```python
from build123d import *

# Parameters (mm, degrees)
F0_R     = 63.5
F0_R_2   = 1.5875
F1_DEPTH = 3.175


with BuildPart() as f1:
    # F0 (on Front) → F1 (new body)
    with BuildSketch(Plane.XZ):
        Circle(F0_R)
        with BuildLine():
            ThreePointArc((-12.832221, -55.690723), (-24.872502, -51.45368), (-35.672091, -44.650021))
            Line((-35.672091, -44.650021), (-8.873024, -9.086223))
            ThreePointArc((-8.873024, -9.086223), (-5.527223, -11.434151), (-1.608887, -12.597678))
            Line((-1.608887, -12.597678), (-12.832221, -55.690723))
        make_face(mode=Mode.SUBTRACT)
        with BuildLine():
            ThreePointArc((-51.541519, -24.689963), (-55.735858, -12.634739), (-57.149977, 0.050731))
            Line((-57.149977, 0.050731), (-12.636135, 1.272042))
            ThreePointArc((-12.636135, 1.272042), (-12.385746, -2.80772), (-10.852385, -6.596645))
            Line((-10.852385, -6.596645), (-51.541519, -24.689963))
        make_face(mode=Mode.SUBTRACT)
        with BuildLine():
            ThreePointArc((35.540001, -44.755232), (24.720355, -51.52695), (12.667607, -55.728397))
            Line((12.667607, -55.728397), (1.571655, -12.602377))
            ThreePointArc((1.571655, -12.602377), (5.493412, -11.450433), (8.846137, -9.112402))
            Line((8.846137, -9.112402), (35.540001, -44.755232))
        make_face(mode=Mode.SUBTRACT)
        with BuildLine():
            ThreePointArc((57.149878, -0.118139), (55.698281, -12.799376), (51.468339, -24.842153))
            Line((51.468339, -24.842153), (10.832846, -6.628684))
            ThreePointArc((10.832846, -6.628684), (12.377396, -2.844306), (12.639839, 1.234699))
            Line((12.639839, 1.234699), (57.149878, -0.118139))
        make_face(mode=Mode.SUBTRACT)
        with BuildLine():
            ThreePointArc((-51.439002, 24.902842), (-44.628976, 35.698417), (-35.592765, 44.713282))
            Line((-35.592765, 44.713282), (-6.883979, 10.672433))
            ThreePointArc((-6.883979, 10.672433), (-9.91755, 7.932982), (-11.923817, 4.371795))
            Line((-11.923817, 4.371795), (-51.439002, 24.902842))
        make_face(mode=Mode.SUBTRACT)
        Circle(F0_R_2, mode=Mode.SUBTRACT)
        with BuildLine():
            ThreePointArc((35.724731, 44.607915), (44.734265, 35.566389), (51.512362, 24.750739))
            Line((51.512362, 24.750739), (11.936683, 4.336543))
            ThreePointArc((11.936683, 4.336543), (9.940948, 7.903642), (6.915484, 10.652046))
            Line((6.915484, 10.652046), (35.724731, 44.607915))
        make_face(mode=Mode.SUBTRACT)
        with BuildLine():
            ThreePointArc((-12.601867, 55.7433), (0.084435, 57.149938), (12.766526, 55.705819))
            Line((12.766526, 55.705819), (4.051954, 12.036265))
            ThreePointArc((4.051954, 12.036265), (0.018763, 12.699986), (-4.016371, 12.048185))
            Line((-4.016371, 12.048185), (-12.601867, 55.7433))
        make_face(mode=Mode.SUBTRACT)
    extrude(amount=F1_DEPTH)


solid = f1.part
```
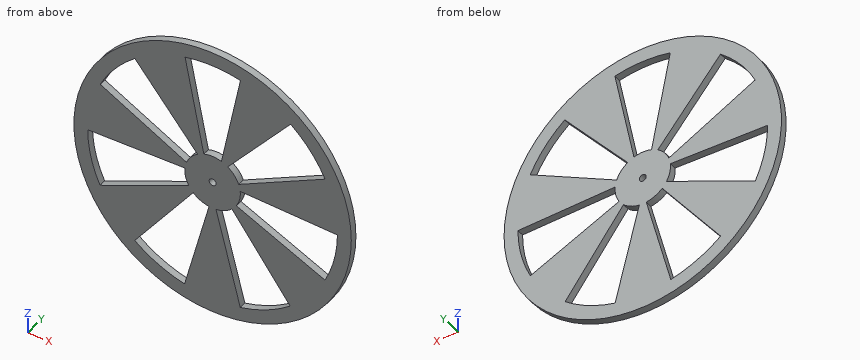
Work out the finished part from the listing and answer in its coordinate system (mm). Round coordinates to 2 decimals unless told otherwise and drop trailing zeros. Write each loop counter-clockwise with the first axis right and the second up, starting at its lowest first coordinate (ties: lowest second). Pieces come first, ordered by that corner, then holes.
1) A cutting plane is placed at B-B on z = 18. Determine the outline of the cut face in (x, y) (3 decimals), and give its area (3 significant figures).
2) A cutting plane is placed at A-A on x = 0. Give the number of separate pieces and of enclosed holes in the cut face, and give its area (3 significant figures).
3) Consider probe 1 along Z at (x, y) = (0, -1); probe 2 along Z at (x, y) = (16.5, -2.9); probe 3 along X at (y, z) = (-2.1, 15). Determine where each line is inside the solid, lowest interval first.
4) A flat-ended cylindrical pin translates along its axis: P1, Ø1, axis at y = -2.5, z = -37.5, coming from the -X side. Find the tip coordinate at first contact, or state that the pin passes through.
5) A cutting plane is placed at D-D on x = -18. Determine the outline of the cut face in (y, z) (3 decimals).
Entries:
1. outline: (-60.895, -3.175) - (-38.153, -3.175) - (-38.153, 0) - (-60.895, 0) - close; (-13.064, -3.175) - (-5.186, -3.175) - (-5.186, 0) - (-13.064, 0) - close; (5.242, -3.175) - (13.15, -3.175) - (13.15, 0) - (5.242, 0) - close; (38.425, -3.175) - (60.895, -3.175) - (60.895, 0) - (38.425, 0) - close
1. area: 194 mm2
2. separate pieces: 3
2. enclosed holes: 0
2. area: 252 mm2
3. probe 1: z = -63.5 to -1.59, 1.59 to 12.7, 57.15 to 63.5
3. probe 2: z = -61.32 to -54.72, -19.33 to -9.17, 1.12 to 6.69, 21.95 to 61.32
3. probe 3: x = -61.7 to -32.38, -10.53 to -4.6, 4.64 to 10.6, 32.61 to 61.7
4. P1: stops at x = -51.61
5. outline: (-3.175, -60.895) - (0, -60.895) - (0, -54.241) - (-3.175, -54.241) - close; (-3.175, -21.198) - (0, -21.198) - (0, -9.775) - (-3.175, -9.775) - close; (-3.175, 1.125) - (0, 1.125) - (0, 7.529) - (-3.175, 7.529) - close; (-3.175, 23.853) - (0, 23.853) - (0, 60.895) - (-3.175, 60.895) - close
